For this review, use the dimensioned drawing (mm, ordinates from the lowest corner) and the shaded views. A direction names the side the tool comes from. Round coordinates to 2 decimals unless told otherwise and drop trailing zeros. Loops run counter-clockwise (first coordinate to the right, second up) from the corner with the lowest first, then second, coordinate; pieces in that order, holes last. Notation, with made-up numbers: (-7.75, 73) - (-0.75, 73) arc R24 cw to (-0.75, 88) - close; hole circle Ø6 at (28, 71.5). An arc over 180 degrees is marked (long way). Answer as CSV lines item,"result". Start each with the question number.
(1) Wall thickness on L1, parallel to X at y = 3, z = 55; L2, parallel to Y at x = 446, z = 15; L3, parallel to Z at x = 350, y = 3: over which ranges is each line inside the solid? List them lowest first.
(2) Consider section B-B (x = 380). Give the boundary of the cut face in (y, z), and give its area (3 significant figures).
(3) For P1, Ø8, axis at x = 191, z = 22, coming from the -Y side; P2, Ø21, axis at x = 430, z = 55, coming from the -Y side; P3, Ø6, axis at x = 323.5, z = 22, coming from the +Y side; P4, Ø4, axis at y = 273, z = 9, coming from the -X side, all flat-tipped, find the tip position at first contact; note any pin that passes through.
(4) Consider section A-A (x = 194). Give the boundary of the cut face in (y, z).
(5) Consider section C-C (y = 203). Give the boundary of the cut face in (x, z), and give its area (3 significant figures).
(6) For the marked faces 1 and 2, list the 3-axis set-ups (+Z, -Z, +X, -X, +Y, -Y) from which the entire face can be reached by the end or side of a thin tool; tool diameter is ignored.
(7) Consider section D-D (x = 278). Give the boundary of the cut face in (y, z).
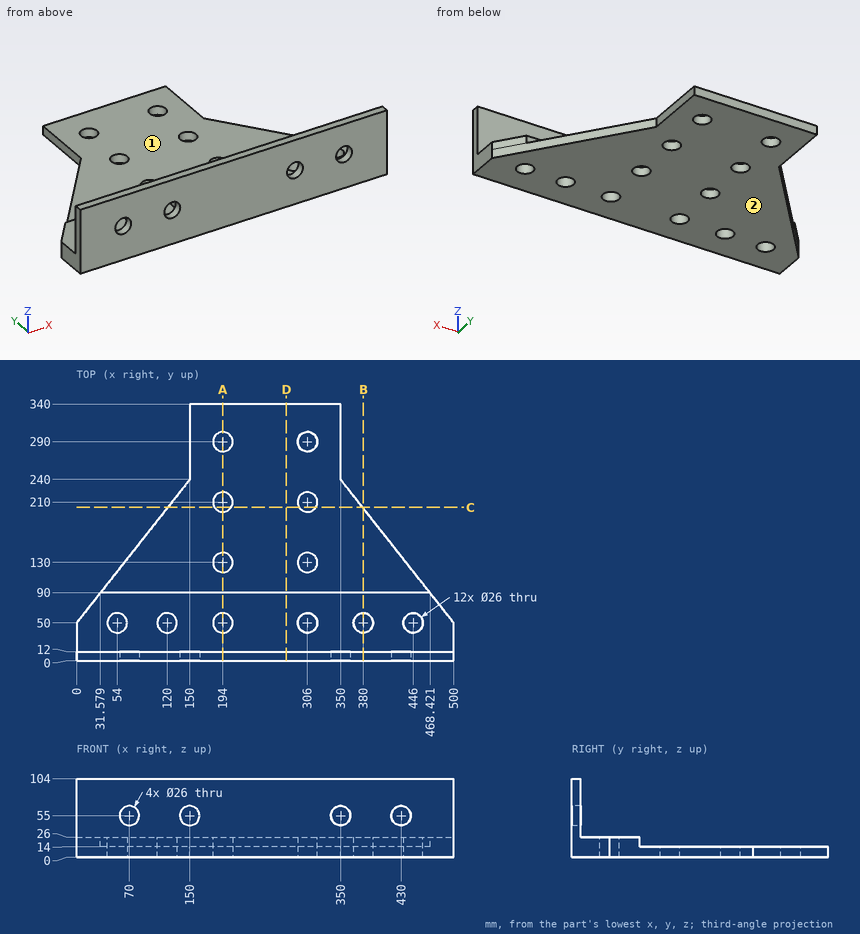
Determined:
1,L1,"x = 0 to 57, 83 to 137, 163 to 337, 363 to 417, 443 to 500"
1,L2,"y = 0 to 37, 63 to 90"
1,L3,"z = 0 to 42, 68 to 104"
2,outline,"(0, 0) - (37, 0) - (37, 26) - (12, 26) - (12, 104) - (0, 104) - close; (63, 0) - (202, 0) - (202, 14) - (90, 14) - (90, 26) - (63, 26) - close"
2,area,"4,170 mm^2"
3,P1,"stops at y = 0"
3,P2,"passes through"
3,P3,"stops at y = 90"
3,P4,"stops at x = 150"
4,outline,"(0, 0) - (37, 0) - (37, 26) - (12, 26) - (12, 104) - (0, 104) - close; (63, 0) - (117, 0) - (117, 14) - (90, 14) - (90, 26) - (63, 26) - close; (143, 0) - (197, 0) - (197, 14) - (143, 14) - close; (223, 0) - (277, 0) - (277, 14) - (223, 14) - close; (303, 0) - (340, 0) - (340, 14) - (303, 14) - close"
5,outline,"(120.79, 0) - (183.05, 0) - (183.05, 14) - (120.79, 14) - close; (204.95, 0) - (295.05, 0) - (295.05, 14) - (204.95, 14) - close; (316.95, 0) - (379.21, 0) - (379.21, 14) - (316.95, 14) - close"
5,area,"3,000 mm^2"
6,face 1,"+Z, +X, -X, +Y"
6,face 2,"-Z, +X, -X, +Y, -Y"
7,outline,"(0, 0) - (340, 0) - (340, 14) - (90, 14) - (90, 26) - (12, 26) - (12, 104) - (0, 104) - close"
